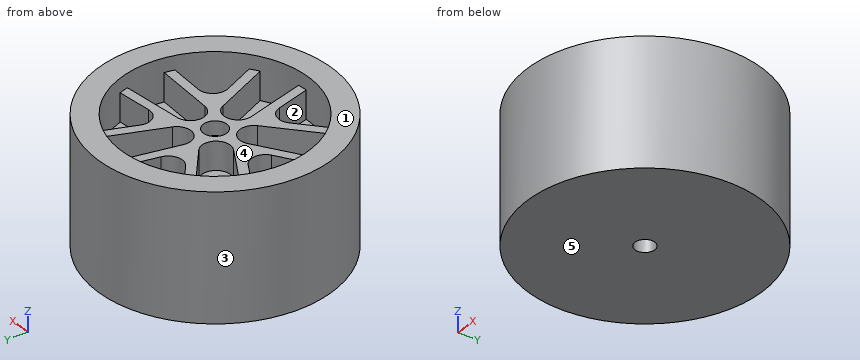
Autodesk Inventor part; units mm, degrees
ref_plane "YZ Plane" through (0, 0, 0) normal (1, 0, 0) x (0, 1, 0)
ref_plane "XZ Plane" through (0, 0, 0) normal (0, 1, 0) x (-1, 0, 0)
ref_plane "XY Plane" through (0, 0, 0) normal (0, 0, 1) x (1, 0, 0)
sketch "草圖1" plane through (0, 0, 0) normal (0, 0, 1) x (1, 0, 0)
  circle A0 centre (0, 0) radius 25
  circle A1 centre (0, 0) radius 2.1
  dimension "d0" = 50
  dimension "d1" = 4.2
extrude "擠出1" add sketch "草圖1" along normal blind 27
sketch "Sketch2" plane through (0, 0, 27) normal (0, 0, 1) x (1, 0, 0)
  circle A0 centre (0, 0) radius 25
  circle A1 centre (0, 0) radius 20
  dimension "d4" = 40
extrude "Extrusion2" cut sketch "Sketch2" against normal blind 3 contours A1
sketch "Sketch4" plane through (0, 0, 24) normal (0, 0, 1) x (1, 0, 0)
  circle A0 centre (0, 0) radius 2.1
extrude "Extrusion3" add sketch "Sketch4" against normal up to surface (24 mm away)
sketch "Sketch5" plane through (0, 0, 24) normal (0, 0, 1) x (1, 0, 0)
  arc A0 (6.7648, 2.9908) -> (6.7648, -2.9908) centre (7, 0) ccw
  circle A1 centre (0, 0) radius 20
  line L0 (19.5959, 4) -> (6.7648, 2.9908)
  line L1 (19.5959, -4) -> (6.7648, -2.9908)
  line L2 (9.8597, 17.4008) -> (4.9348, 5.5095)
  arc A2 (-0.754, 7.3579) -> (4.9348, 5.5095) centre (2.1631, 6.6574) ccw
  line L3 (2.2512, 19.8729) -> (-0.754, 7.3579)
  line L4 (-13.5023, 14.7543) -> (-3.7149, 6.3958)
  arc A3 (-7.2307, 1.5566) -> (-3.7149, 6.3958) centre (-5.6631, 4.1145) ccw
  line L5 (-18.2046, 8.2821) -> (-7.2307, 1.5566)
  line L6 (-18.2046, -8.2821) -> (-7.2307, -1.5566)
  arc A4 (-3.7149, -6.3958) -> (-7.2307, -1.5566) centre (-5.6631, -4.1145) ccw
  line L7 (-13.5023, -14.7543) -> (-3.7149, -6.3958)
  line L8 (2.2512, -19.8729) -> (-0.754, -7.3579)
  arc A5 (4.9348, -5.5095) -> (-0.754, -7.3579) centre (2.1631, -6.6574) ccw
  line L9 (9.8597, -17.4008) -> (4.9348, -5.5095)
  line L10 (11.7075, 16.6355) -> (8.7645, 9.5294)
  line L11 (19.4391, 5.9938) -> (11.7714, 5.3907)
  line L12 (19.0893, -5.9663) -> (19.4391, -5.9938)
  arc A6 (8.7645, 9.5294) -> (11.7714, 5.3907) centre (11.5361, 8.3815) ccw
  circle A7 centre (0, 0) radius 20
  line L13 (0.3065, 20.3399) -> (-1.4893, 12.8611)
  arc A8 (-6.3547, 11.2802) -> (-1.4893, 12.8611) centre (-4.4064, 13.5616) ccw
  line L14 (-12.2035, 16.2751) -> (-6.3547, 11.2802)
  line L15 (-19.2496, 6.5769) -> (-12.6918, 2.5578)
  arc A9 (-12.6918, -2.5578) -> (-12.6918, 2.5578) centre (-14.2595, 0) ccw
  line L16 (-19.2496, -6.5769) -> (-12.6918, -2.5578)
  line L17 (-12.2035, -16.2751) -> (-6.3547, -11.2802)
  arc A10 (-1.4893, -12.8611) -> (-6.3547, -11.2802) centre (-4.4064, -13.5616) ccw
  line L18 (0.3065, -20.3399) -> (-1.4893, -12.8611)
  line L19 (11.7075, -16.6355) -> (8.7645, -9.5294)
  arc A11 (11.7714, -5.3907) -> (8.7645, -9.5294) centre (11.5361, -8.3815) ccw
  line L20 (19.4391, -5.9938) -> (11.7714, -5.3907)
  point P0 (19.0893, 5.9663)
  point P1 (11.5732, 16.3113)
  point P2 (11.5732, -16.3113)
  point P3 (-11.9367, -16.0473)
  point P4 (0.2246, -19.9987)
  point P5 (-18.9505, 6.3936)
  point P6 (-18.9505, -6.3936)
  point P7 (0.2246, 19.9987)
  point P8 (-11.9367, 16.0473)
  dimension "d9" = 6
  dimension "d12" = 360
  dimension "d14" = 2
  dimension "d15" = 2
  dimension "d16" = 3
  dimension "d19" = 360
extrude "Extrusion4" cut sketch "Sketch5" against normal blind 6 contours L0 A1 L1 A0 | L11 A6 L10 A1 | A1 L19 A11 L20 | L2 A2 L3 A1 | A1 L8 A5 L9 | L13 A8 L14 A1 | A1 L17 A10 L18 | L4 A3 L5 A1 | A1 L6 A4 L7 | L15 A9 L16 A1
sketch "Sketch9" plane through (0, 0, 0) normal (0, 0, -1) x (-1, 0, 0)
  circle A0 centre (0, 0) radius 2.1
  dimension "d38" = 4.2
extrude "Extrusion7" cut sketch "Sketch9" against normal blind 18
sketch "Sketch10" plane through (0, 0, 24) normal (0, 0, 1) x (1, 0, 0)
  circle A0 centre (0, 0) radius 2.1
  circle A1 centre (0, 0) radius 2.5
  dimension "d41" = 5
extrude "Extrusion8" cut sketch "Sketch10" against normal blind 3 contours A0 | A1
properties part number "前輪 改"
The listing builds one solid part. Answer for the finished solid, in the listing's coordinates (mm). Face numbers are marked on the shaded views. A direction names the side the tool comes from. Coordinates: 2 decimals unless noted, no trailing zeros. Loops run counter-clockwise (first coordinate to the right, second up) from the corner with the lowest first, then second, coordinate; pieces in that order, holes last. Notation, with made-up numbers: (39.5, -6) -> (66.5, -6) arc R33 ccw to (66.5, 33) -> close; hole circle Ø8 at (29, 62). An arc over 180 degrees is marked (long way). Write item = value, one per line. Start each with the question number.
1) A tool of negligible diameter and unlimited length cuts with its end or side. For the marked faces 1 and 2, from which of +Z, -Z, +X, -X, +Y, -Y can it reach the whole face along a straight path? Write none if from no direction.
2) A cutting plane is placed at B-B (z = 5). Give the vertices of the cut face in (x, y).
3) Straight lines are drawn through the part: line 1 (Y direction, x = 0, z = 9.75); line 2 (Z direction, x = -8, y = -13); line 3 (Z direction, x = -9.5, y = -13). For each, find the intervals that lie inside material, in ascending order. Write a range as from..to.
4) A cutting plane is placed at A-A (y = 0). Give the vertices of the cut face in (x, z), then the cut area to 3 significant figures.
5) A cutting plane is placed at D-D (y = 21). Give the vertices of the cut face in (x, z).
6) Given pin 1 Ø4 at (x, z) = (2, 18.5) entering from -Y; pin 2 Ø5 at (x, y) = (-6, -1) entering from +Z; pin 3 Ø1 at (x, y) = (-4, 12.5) entering from +Z; pin 4 Ø12 at (y, z) = (2, 15) entering from +X, each flat-ended and moving along its own axis, determine where each tip first touches the part or whether it passes through.
7) A cutting plane is placed at C-C (x = -5.5). Give the vertices of the cut face in (y, z), then the cut area to 3 significant figures.
8) The mould has two halves that part along X. Classify the marked faces 3, 4 and 5: released by +X, released by -X, zero draft, split by the parting line, or undercut.
Responses:
q1.face_1 = +Z, +X, -X, +Y, -Y
q1.face_2 = +Z
q2.outline = circle Ø50 at (0, 0); hole circle Ø4.2 at (0, 0)
q3.line_1 = -25..-2.1, 2.1..25
q3.line_2 = 0..18
q3.line_3 = 0..24
q4.outline = (-25, 0) -> (-2.1, 0) -> (-2.1, 18) -> (2.1, 18) -> (2.1, 0) -> (25, 0) -> (25, 27) -> (20, 27) -> (20, 18) -> (4, 18) -> (4, 24) -> (2.5, 24) -> (2.5, 21) -> (-2.5, 21) -> (-2.5, 24) -> (-11.26, 24) -> (-11.26, 18) -> (-20, 18) -> (-20, 27) -> (-25, 27) -> close
q4.area = 991 mm²
q5.outline = (-13.56, 0) -> (13.56, 0) -> (13.56, 27) -> (-13.56, 27) -> close
q6.pin_1 = -25
q6.pin_2 = 24
q6.pin_3 = 18
q6.pin_4 = 25
q7.outline = (-24.39, 0) -> (24.39, 0) -> (24.39, 27) -> (19.23, 27) -> (19.23, 18) -> (10.77, 18) -> (10.77, 24) -> (7.92, 24) -> (7.92, 18) -> (1.12, 18) -> (1.12, 24) -> (-1.12, 24) -> (-1.12, 18) -> (-7.92, 18) -> (-7.92, 24) -> (-10.77, 24) -> (-10.77, 18) -> (-19.23, 18) -> (-19.23, 27) -> (-24.39, 27) -> close
q7.area = 1,020 mm²
q8.face_3 = split by the parting line
q8.face_4 = undercut
q8.face_5 = zero draft
